Model file for the job. Use its own axes, mm. Face numbers are marked on the shaded views. A direction names the side the tool comes from. Give positions to 0.01 mm unless a question says otherwise; leave off trailing zeros. Write each loop counter-clockwise with the first axis right and the second up, starting at its lowest first coordinate (ties: lowest second). Pieces come first, ordered by that corner, then holes.
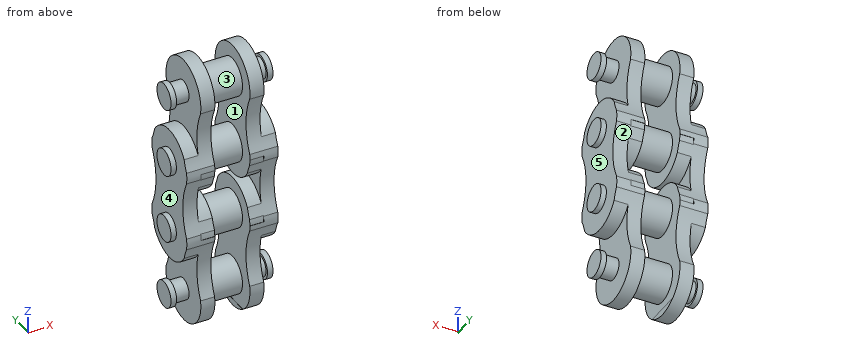
```python
from build123d import *

# Parameters (mm, degrees)
BOSS_EXTRUDE1_DEPTH      = 6.19125
BOSS_EXTRUDE1_DEPTH_BACK = 6.19125
CUT_EXTRUDE1_DEPTH       = 1.905
CUT_EXTRUDE1_DEPTH_BACK  = 1.905
CUT_EXTRUDE2_DEPTH       = 1.905
CUT_EXTRUDE2_DEPTH_BACK  = 1.905
CUT_EXTRUDE3_DEPTH       = 4.26085
CUT_EXTRUDE3_DEPTH_BACK  = 4.26085
CUT_EXTRUDE4_DEPTH       = 2.38125
CUT_EXTRUDE4_DEPTH_BACK  = 2.38125
SKETCH5_W                = 41.063333333
SKETCH5_H                = 17.78
CUT_EXTRUDE5_DEPTH       = 2.35585
CUT_EXTRUDE5_DEPTH_BACK  = 2.35585
SKETCH7_W                = 28.575
SKETCH7_H                = 17.78


with BuildPart() as part:
    # Sketch1 → Boss-Extrude1 (new, two sides: drawn at the far end of the back side and taken through both)
    with BuildSketch(Plane(origin=(0, 0, 0), x_dir=(0, 0, -1), z_dir=(1, 0, 0)).offset(-BOSS_EXTRUDE1_DEPTH_BACK)):
        with BuildLine():
            ThreePointArc((0.77186615, 4.377470462), (-4.445, 0), (0.77186615, -4.377470462))
            ThreePointArc((0.77186615, -4.377470462), (4.7625, -3.431458218), (8.75313385, -4.377470462))
            ThreePointArc((8.75313385, -4.377470462), (9.525, -4.445), (10.29686615, -4.377470462))
            ThreePointArc((10.29686615, -4.377470462), (14.2875, -3.431458218), (18.27813385, -4.377470462))
            ThreePointArc((18.27813385, -4.377470462), (19.05, -4.445), (19.82186615, -4.377470462))
            ThreePointArc((19.82186615, -4.377470462), (23.8125, -3.431458218), (27.80313385, -4.377470462))
            ThreePointArc((27.80313385, -4.377470462), (33.02, 0), (27.80313385, 4.377470462))
            ThreePointArc((27.80313385, 4.377470462), (23.8125, 3.431458218), (19.82186615, 4.377470462))
            ThreePointArc((19.82186615, 4.377470462), (19.05, 4.445), (18.27813385, 4.377470462))
            ThreePointArc((18.27813385, 4.377470462), (14.2875, 3.431458218), (10.29686615, 4.377470462))
            ThreePointArc((10.29686615, 4.377470462), (9.525, 4.445), (8.75313385, 4.377470462))
            ThreePointArc((8.75313385, 4.377470462), (4.7625, 3.431458218), (0.77186615, 4.377470462))
        make_face()
    extrude(amount=BOSS_EXTRUDE1_DEPTH + BOSS_EXTRUDE1_DEPTH_BACK)

    # Sketch2 → Cut-Extrude1 (cut, two sides: drawn at the far end of the back side and taken through both)
    with BuildSketch(Plane(origin=(6.19125, 0, 0), x_dir=(0, 0, -1), z_dir=(1, 0, 0)).offset(-CUT_EXTRUDE1_DEPTH_BACK)):
        with BuildLine():
            Line((-8.89, -4.5466), (9.525, -4.5466))
            Line((9.525, -4.5466), (9.525, -4.445))
            ThreePointArc((9.525, -4.445), (5.08, 0), (9.525, 4.445))
            Line((9.525, 4.445), (9.525, 4.5466))
            Line((9.525, 4.5466), (19.05, 4.5466))
            Line((19.05, 4.5466), (19.05, 4.445))
            ThreePointArc((19.05, 4.445), (23.495, 0), (19.05, -4.445))
            Line((19.05, -4.445), (19.05, -4.5466))
            Line((19.05, -4.5466), (38.1, -4.5466))
            Line((38.1, -4.5466), (38.1, 13.4366))
            Line((38.1, 13.4366), (-8.89, 13.4366))
            Line((-8.89, 13.4366), (-8.89, -4.5466))
        make_face()
    extrude(amount=CUT_EXTRUDE1_DEPTH + CUT_EXTRUDE1_DEPTH_BACK, mode=Mode.SUBTRACT)

    # Sketch3 → Cut-Extrude2 (cut, two sides: drawn at the far end of the back side and taken through both)
    with BuildSketch(Plane.ZY.offset(6.19125).offset(-CUT_EXTRUDE2_DEPTH_BACK)):
        with BuildLine():
            Line((-38.1, -4.5466), (-19.05, -4.5466))
            Line((-19.05, -4.5466), (-19.05, -4.445))
            ThreePointArc((-19.05, -4.445), (-23.495, 0), (-19.05, 4.445))
            Line((-19.05, 4.445), (-19.05, 4.5466))
            Line((-19.05, 4.5466), (-9.525, 4.5466))
            Line((-9.525, 4.5466), (-9.525, 4.445))
            ThreePointArc((-9.525, 4.445), (-5.08, 0), (-9.525, -4.445))
            Line((-9.525, -4.445), (-9.525, -4.5466))
            Line((-9.525, -4.5466), (8.89, -4.5466))
            Line((8.89, -4.5466), (8.89, 13.4366))
            Line((8.89, 13.4366), (-38.1, 13.4366))
            Line((-38.1, 13.4366), (-38.1, -4.5466))
        make_face()
    extrude(amount=CUT_EXTRUDE2_DEPTH + CUT_EXTRUDE2_DEPTH_BACK, mode=Mode.SUBTRACT)

    # Sketch4 → Cut-Extrude3 (cut, two sides: drawn at the far end of the back side and taken through both)
    with BuildSketch(Plane(origin=(0, 0, 0), x_dir=(0, 0, -1), z_dir=(1, 0, 0)).offset(-CUT_EXTRUDE3_DEPTH_BACK)):
        with BuildLine():
            Line((9.525, -4.4958), (19.05, -4.4958))
            Line((19.05, -4.4958), (19.05, -4.4196))
            ThreePointArc((19.05, -4.4196), (14.6304, 0), (19.05, 4.4196))
            Line((19.05, 4.4196), (19.05, 4.4958))
            Line((19.05, 4.4958), (9.525, 4.4958))
            Line((9.525, 4.4958), (9.525, 4.4196))
            ThreePointArc((9.525, 4.4196), (13.9446, 0), (9.525, -4.4196))
            Line((9.525, -4.4196), (9.525, -4.4958))
        make_face()
    extrude(amount=CUT_EXTRUDE3_DEPTH + CUT_EXTRUDE3_DEPTH_BACK, mode=Mode.SUBTRACT)

    # Sketch5 → Cut-Extrude4 (cut, two sides: drawn at the far end of the back side and taken through both)
    with BuildSketch(Plane(origin=(0, 0, 0), x_dir=(0, 0, -1), z_dir=(1, 0, 0)).offset(-CUT_EXTRUDE4_DEPTH_BACK)):
        with Locations((11.641666667, 0)):
            Rectangle(SKETCH5_W, SKETCH5_H)
    extrude(amount=CUT_EXTRUDE4_DEPTH + CUT_EXTRUDE4_DEPTH_BACK, mode=Mode.SUBTRACT)

    # Sketch6 → Revolve1 (revolve)
    with BuildSketch(Plane(origin=(0, 0, 0), x_dir=(1, 0, 0), z_dir=(0, 1, 0)), mode=Mode.PRIVATE) as revolve1_sk:
        Polygon((-6.9215, 0), (-6.9215, 1.7907), (-6.16585, 1.7907), (-6.16585, 1.43256), (-2.40665, 1.43256), (-2.40665, 2.54), (2.40665, 2.54), (2.40665, 1.43256), (6.16585, 1.43256), (6.16585, 1.7907), (6.9215, 1.7907), (6.9215, 0), align=None)
    revolve(revolve1_sk.sketch.rotate(Axis((6.9215, 0, 0), (-1, 0, 0)), 180), axis=Axis((6.9215, 0, 0), (-1, 0, 0)))

    # Sketch7 → Cut-Extrude5 (cut, two sides: drawn at the far end of the back side and taken through both)
    with BuildSketch(Plane(origin=(0, 0, 0), x_dir=(0, 0, -1), z_dir=(1, 0, 0)).offset(-CUT_EXTRUDE5_DEPTH_BACK)):
        with Locations((33.2105, 0)):
            Rectangle(SKETCH7_W, SKETCH7_H)
    extrude(amount=CUT_EXTRUDE5_DEPTH + CUT_EXTRUDE5_DEPTH_BACK, mode=Mode.SUBTRACT)

    # Sketch8 → Revolve2 (revolve)
    with BuildSketch(Plane(origin=(0, 0, 0), x_dir=(1, 0, 0), z_dir=(0, 1, 0)), mode=Mode.PRIVATE) as revolve2_sk:
        Polygon((-6.9215, 28.575), (-6.9215, 30.3657), (-6.16585, 30.3657), (-6.16585, 30.00756), (-2.40665, 30.00756), (-2.40665, 31.115), (2.40665, 31.115), (2.40665, 30.00756), (6.16585, 30.00756), (6.16585, 30.3657), (6.9215, 30.3657), (6.9215, 28.575), align=None)
    revolve(revolve2_sk.sketch.rotate(Axis((6.9215, 0, -28.575), (-1, 0, 0)), 180), axis=Axis((6.9215, 0, -28.575), (-1, 0, 0)))

    # Sketch9 → Revolve3 (revolve)
    with BuildSketch(Plane(origin=(0, 0, 0), x_dir=(1, 0, 0), z_dir=(0, 1, 0)), mode=Mode.PRIVATE) as revolve3_sk:
        Polygon((-6.9215, 19.05), (-6.9215, 20.8407), (-6.16585, 20.8407), (-6.16585, 20.48256), (-2.40665, 20.48256), (-2.40665, 21.59), (2.40665, 21.59), (2.40665, 20.48256), (6.16585, 20.48256), (6.16585, 20.8407), (6.9215, 20.8407), (6.9215, 19.05), align=None)
    revolve(revolve3_sk.sketch.rotate(Axis((6.9215, 0, -19.05), (-1, 0, 0)), 180), axis=Axis((6.9215, 0, -19.05), (-1, 0, 0)))

    # Sketch10 → Revolve4 (revolve)
    with BuildSketch(Plane(origin=(0, 0, 0), x_dir=(1, 0, 0), z_dir=(0, 1, 0)), mode=Mode.PRIVATE) as revolve4_sk:
        Polygon((-6.9215, 9.525), (-6.9215, 11.3157), (-6.16585, 11.3157), (-6.16585, 10.95756), (-2.40665, 10.95756), (-2.40665, 12.065), (2.40665, 12.065), (2.40665, 10.95756), (6.16585, 10.95756), (6.16585, 11.3157), (6.9215, 11.3157), (6.9215, 9.525), align=None)
    revolve(revolve4_sk.sketch.rotate(Axis((6.9215, 0, -9.525), (-1, 0, 0)), 180), axis=Axis((6.9215, 0, -9.525), (-1, 0, 0)))


solid = part.part
```
1. Probe probe 1 along X at (y, z) = (-1.75, -28.5); probe 2 along Z at (x, y) = (-0.5, 1.5); probe 3 along Z at (x, y) = (-4.75, -0.5). List the from-to ranges inside material, lowest first.
Calculated:
probe 1: x = -6.92 to -6.17, -4.29 to 4.29, 6.17 to 6.92
probe 2: z = -30.62 to -26.53, -21.1 to -17, -11.57 to -7.48, -2.05 to 2.05
probe 3: z = -29.92 to -27.23, -23.47 to -5.11, -1.34 to 1.34
2. Pull direction X, two halves, no side cores. Call the marked faces 3, 4 and 5: +X half, -X half, draft (parallel to the pull), parting line (faces both ways), or undercut.
Calculated:
face 3: undercut
face 4: -X half
face 5: +X half
3. Which spindle directions (+Z, -Z, +X, -X, +Y, -Y) get a long thin tool onto all of the face, cutting with end or side? Do the marked faces 1 and 2. Say none if no direction does.
Calculated:
face 1: none
face 2: +X, -X, +Y
4. Slice it at C-C, the plane z = -15.5. Write the cut outline in (x, y), and give its area (3 significant figures).
Calculated:
outline: (-6.19, -3.51) - (-4.26, -3.51) - (-4.26, -2.63) - (-2.38, -2.63) - (-2.38, 2.63) - (-4.26, 2.63) - (-4.26, 3.51) - (-6.19, 3.51) - close; (2.38, -2.63) - (4.26, -2.63) - (4.26, -3.51) - (6.19, -3.51) - (6.19, 3.51) - (4.26, 3.51) - (4.26, 2.63) - (2.38, 2.63) - close
area: 46.9 mm2
5. Slice it at B-B, the plane x = -5.5. State how many separate pieces and enclosed holes the cut face has, and give its area (3 significant figures).
Calculated:
separate pieces: 3
enclosed holes: 0
area: 148 mm2
6. Pin check, flat tips, straight feed: P1, Ø2, axis at y = -1.5, z = -27.5, coming from the -X side; P2, Ø0.9, axis at y = 1, z = -32.5, coming from the -X side; P3, Ø1.5, axis at y = -3.5, z = -22.5, coming from the -X side; P4, Ø3, axis at y = -2.5, z = -12, coming from the +X side. Stop position of each tip, or through.
Calculated:
P1: stops at x = -6.92
P2: stops at x = -4.29
P3: stops at x = -6.19
P4: stops at x = 6.19
